Read the model definition and answer for the solid it produces. Units are mm, in the model's axes. Coordinates: 2 decimals unless noted, no trailing zeros. Write each loop counter-clockwise with the first axis right and the second up, starting at its lowest first coordinate (ties: lowest second). Pieces come first, ordered by that corner, then holes.
Item 1: Section B-B (x = 33) is taken. Give the vertices of the cut face in (y, z), then the cut area to 3 significant figures.
Item 2: Straight lines are drawn through the part: probe 1 along Z at (x, y) = (74, 79.25); probe 2 along Z at (x, y) = (8, 85.75); probe 3 along Y at (x, z) = (66, 15). For each, find the intervals that lie inside material, in ascending order.
Item 3: Each of these flat-tipped pins is pushed along its axis until it touches: P1, Ø0.9, axis at y = 86, z = 22, coming from the -X side; P2, Ø1.1, axis at x = -3.5, z = 15, coming from the +Y side; P3, Ø1.5, axis at y = 84.5, z = 18.5, coming from the +X side; P4, Ø0.7, axis at x = 36, z = 23, coming from the +Y side. Where does it stop, or does it pass through?
Item 4: Section A-A (x = 17) is taken. Give the vertices of the cut face in (y, z).
from build123d import *

# Parameters (mm, degrees)
BOSS_EXTRUDE1_DEPTH = 140
SKETCH1_5_R         = 0.75
BOSS_EXTRUDE2_DEPTH = 5
SKETCH2_R           = 0.9
SKETCH2_R_2         = 0.75
CUT_EXTRUDE1_DEPTH  = 6
SKETCH3_W           = 0.25
SKETCH3_H           = 1
CUT_EXTRUDE2_DEPTH  = 171.461242575
SKETCH4_W           = 10
SKETCH4_H           = 2.25
CUT_EXTRUDE3_DEPTH  = 86.659037056
SKETCH6_W           = 10
SKETCH6_H           = 2.25
CUT_EXTRUDE4_DEPTH  = 86.755295051
BOSS_EXTRUDE3_REACH = 87.755
SKETCH7_W           = 3
SKETCH7_H           = 2.25
SKETCH8_W           = 3
SKETCH8_H           = 2.25
BOSS_EXTRUDE4_DEPTH = 1.75


with BuildPart() as part:
    # Sketch1 → Boss-Extrude1 (new body)
    with BuildSketch(Plane(origin=(-58.146340827, 0, 0), x_dir=(0, 0, -1), z_dir=(1, 0, 0))):
        Polygon((-20.52887033, 86.340306989), (-21.62887033, 86.340306989), (-21.62887033, 85.490306989), (-21.27887033, 85.490306989), (-21.27887033, 84.590306989), (-23.52887033, 84.590306989), (-23.52887033, 85.490306989), (-22.92887033, 85.490306989), (-22.92887033, 86.340306989), (-24.02887033, 86.340306989), (-24.02887033, 76.840306989), (-13.52887033, 76.840306989), (-13.52887033, 79.340306989), (-14.62887033, 79.340306989), (-14.62887033, 78.490306989), (-14.27887033, 78.490306989), (-14.27887033, 77.590306989), (-16.52887033, 77.590306989), (-16.52887033, 78.490306989), (-15.92887033, 78.490306989), (-15.92887033, 79.340306989), (-17.02887033, 79.340306989), (-17.02887033, 80.340306989), (-20.52887033, 80.340306989), align=None)
    extrude(amount=BOSS_EXTRUDE1_DEPTH)

    # Sketch1<5> → Boss-Extrude2 (add)
    with BuildSketch(Plane(origin=(-58.146340827, 0, 0), x_dir=(0, 0, -1), z_dir=(1, 0, 0))):
        with Locations((-22.27887033, 82.090306989)):
            Circle(SKETCH1_5_R)
        with Locations((-18.77887033, 78.590306989)):
            Circle(SKETCH1_5_R)
    extrude(amount=-BOSS_EXTRUDE2_DEPTH)

    # Sketch2 → Cut-Extrude1 (cut)
    with BuildSketch(Plane(origin=(81.853659173, 0, 0), x_dir=(0, 0, -1), z_dir=(1, 0, 0))):
        with Locations((-22.27887033, 82.090306989)):
            Circle(SKETCH2_R)
        with Locations((-22.27887033, 82.090306989)):
            Circle(SKETCH2_R_2, mode=Mode.SUBTRACT)
        with Locations((-22.27887033, 82.090306989)):
            Circle(SKETCH2_R_2)
        with Locations((-18.77887033, 78.590306989)):
            Circle(SKETCH2_R)
        with Locations((-18.77887033, 78.590306989)):
            Circle(SKETCH2_R_2, mode=Mode.SUBTRACT)
        with Locations((-18.77887033, 78.590306989)):
            Circle(SKETCH2_R_2)
    extrude(amount=-CUT_EXTRUDE1_DEPTH, mode=Mode.SUBTRACT)

    # Sketch3 → Cut-Extrude2 (cut, through all)
    with BuildSketch(Plane(origin=(81.853659173, 0, 0), x_dir=(0, 0, -1), z_dir=(1, 0, 0))):
        with Locations((-17.15387033, 79.840306989)):
            Rectangle(SKETCH3_W, SKETCH3_H)
    extrude(amount=-CUT_EXTRUDE2_DEPTH, mode=Mode.SUBTRACT)

    # Sketch4 → Cut-Extrude3 (cut, through all)
    with BuildSketch(Plane(origin=(0, 84.590306989, 0), x_dir=(1, 0, 0), z_dir=(0, 1, 0))):
        with Locations((73.853659173, -22.40387033)):
            Rectangle(SKETCH4_W, SKETCH4_H)
        with Locations((33.853659173, -22.40387033)):
            Rectangle(SKETCH4_W, SKETCH4_H)
        with Locations((-6.146340827, -22.40387033)):
            Rectangle(SKETCH4_W, SKETCH4_H)
        with Locations((-46.146340827, -22.40387033)):
            Rectangle(SKETCH4_W, SKETCH4_H)
    extrude(amount=CUT_EXTRUDE3_DEPTH, mode=Mode.SUBTRACT)

    # Sketch6 → Cut-Extrude4 (cut, through all)
    with BuildSketch(Plane(origin=(0, 77.590306989, 0), x_dir=(1, 0, 0), z_dir=(0, 1, 0))):
        with Locations((73.853659173, -15.40387033)):
            Rectangle(SKETCH6_W, SKETCH6_H)
        with Locations((33.853659173, -15.40387033)):
            Rectangle(SKETCH6_W, SKETCH6_H)
        with Locations((-6.146340827, -15.40387033)):
            Rectangle(SKETCH6_W, SKETCH6_H)
        with Locations((-46.146340827, -15.40387033)):
            Rectangle(SKETCH6_W, SKETCH6_H)
    extrude(amount=CUT_EXTRUDE4_DEPTH, mode=Mode.SUBTRACT)

    # Boss-Extrude3: up to this face of the body (flat: up to its plane)
    boss_extrude3_end = Plane(part.part.faces().sort_by_distance((11.653659173, 79.340306989, 14.04137033))[0])
    # Sketch7 → Boss-Extrude3 (add, up to the picked face)
    with BuildSketch(Plane(origin=(0, 77.590306989, 0), x_dir=(1, 0, 0), z_dir=(0, 1, 0)), mode=Mode.PRIVATE) as boss_extrude3_sk1:
        with Locations((-55.646340827, -15.40387033)):
            Rectangle(SKETCH7_W, SKETCH7_H)
    boss_extrude3_tool1 = split(extrude(boss_extrude3_sk1.sketch, amount=BOSS_EXTRUDE3_REACH, mode=Mode.PRIVATE), bisect_by=boss_extrude3_end, keep=Keep.BOTH, mode=Mode.PRIVATE)
    # Sketch7 → Boss-Extrude3 (add, up to the picked face)
    with BuildSketch(Plane(origin=(0, 77.590306989, 0), x_dir=(1, 0, 0), z_dir=(0, 1, 0)), mode=Mode.PRIVATE) as boss_extrude3_sk2:
        with Locations((-15.646340827, -15.40387033)):
            Rectangle(SKETCH7_W, SKETCH7_H)
    boss_extrude3_tool2 = split(extrude(boss_extrude3_sk2.sketch, amount=BOSS_EXTRUDE3_REACH, mode=Mode.PRIVATE), bisect_by=boss_extrude3_end, keep=Keep.BOTH, mode=Mode.PRIVATE)
    # Sketch7 → Boss-Extrude3 (add, up to the picked face)
    with BuildSketch(Plane(origin=(0, 77.590306989, 0), x_dir=(1, 0, 0), z_dir=(0, 1, 0)), mode=Mode.PRIVATE) as boss_extrude3_sk3:
        with Locations((24.353659173, -15.40387033)):
            Rectangle(SKETCH7_W, SKETCH7_H)
    boss_extrude3_tool3 = split(extrude(boss_extrude3_sk3.sketch, amount=BOSS_EXTRUDE3_REACH, mode=Mode.PRIVATE), bisect_by=boss_extrude3_end, keep=Keep.BOTH, mode=Mode.PRIVATE)
    # Sketch7 → Boss-Extrude3 (add, up to the picked face)
    with BuildSketch(Plane(origin=(0, 77.590306989, 0), x_dir=(1, 0, 0), z_dir=(0, 1, 0)), mode=Mode.PRIVATE) as boss_extrude3_sk4:
        with Locations((64.353659173, -15.40387033)):
            Rectangle(SKETCH7_W, SKETCH7_H)
    boss_extrude3_tool4 = split(extrude(boss_extrude3_sk4.sketch, amount=BOSS_EXTRUDE3_REACH, mode=Mode.PRIVATE), bisect_by=boss_extrude3_end, keep=Keep.BOTH, mode=Mode.PRIVATE)
    add(boss_extrude3_tool1.solids().sort_by(Axis((-55.646341, 77.590307, 15.40387), (0, 1, 0)))[0])
    add(boss_extrude3_tool2.solids().sort_by(Axis((-15.646341, 77.590307, 15.40387), (0, 1, 0)))[0])
    add(boss_extrude3_tool3.solids().sort_by(Axis((24.353659, 77.590307, 15.40387), (0, 1, 0)))[0])
    add(boss_extrude3_tool4.solids().sort_by(Axis((64.353659, 77.590307, 15.40387), (0, 1, 0)))[0])

    # Sketch8 → Boss-Extrude4 (add)
    with BuildSketch(Plane(origin=(0, 84.590306989, 0), x_dir=(1, 0, 0), z_dir=(0, 1, 0))):
        with Locations((-55.646340827, -22.40387033)):
            Rectangle(SKETCH8_W, SKETCH8_H)
        with Locations((-15.646340827, -22.40387033)):
            Rectangle(SKETCH8_W, SKETCH8_H)
        with Locations((24.353659173, -22.40387033)):
            Rectangle(SKETCH8_W, SKETCH8_H)
        with Locations((64.353659173, -22.40387033)):
            Rectangle(SKETCH8_W, SKETCH8_H)
    extrude(amount=BOSS_EXTRUDE4_DEPTH)


solid = part.part
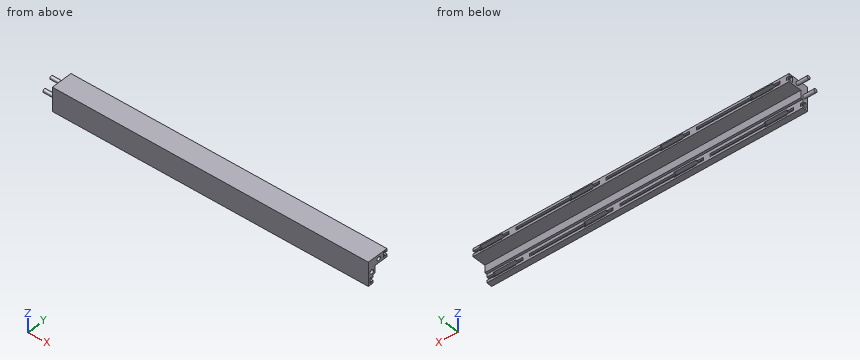
Established:
1. outline: (76.84, 13.53) - (79.34, 13.53) - (79.34, 14.28) - (77.59, 14.28) - (77.59, 16.53) - (79.34, 16.53) - (79.34, 17.28) - (80.34, 17.28) - (80.34, 20.53) - (86.34, 20.53) - (86.34, 21.28) - (84.59, 21.28) - (84.59, 23.53) - (86.34, 23.53) - (86.34, 24.03) - (76.84, 24.03) - close
1. area: 46.1 mm2
2. probe 1: z = 13.53 to 14.28, 16.53 to 24.03
2. probe 2: z = 20.53 to 21.63, 22.93 to 24.03
2. probe 3: y = 76.84 to 77.59
3. P1: stops at x = -58.15
3. P2: stops at y = 77.59
3. P3: passes through
3. P4: stops at y = 84.59
4. outline: (76.84, 13.53) - (79.34, 13.53) - (79.34, 14.63) - (78.49, 14.63) - (78.49, 14.28) - (77.59, 14.28) - (77.59, 16.53) - (78.49, 16.53) - (78.49, 15.93) - (79.34, 15.93) - (79.34, 17.28) - (80.34, 17.28) - (80.34, 20.53) - (86.34, 20.53) - (86.34, 21.63) - (85.49, 21.63) - (85.49, 21.28) - (84.59, 21.28) - (84.59, 23.53) - (85.49, 23.53) - (85.49, 22.93) - (86.34, 22.93) - (86.34, 24.03) - (76.84, 24.03) - close
